from build123d import *

# Parameters (mm, degrees)
SKETCH_1_R          = 2.75
EXTRUDE_1_DEPTH     = 10
CUT_EXTRUDE_1_REACH = 38.009
SKETCH_3_R          = 2.25
SKETCH_3_3_R        = 1.65
CUT_EXTRUDE_2_DEPTH = 37.00893353
FILLET_1_R          = 1
FILLET_2_R          = 0.5
CHAMFER_1_SIZE      = 0.5


with BuildPart() as part:
    # 草图1 → 凸台-拉伸1 (new body)
    with BuildSketch(Plane(origin=(0, 0, 0), x_dir=(1, 0, 0), z_dir=(0, 1, 0))):
        with BuildLine():
            ThreePointArc((5.025690834, 18.234375), (-0.716951035, 21.453070806), (-5.432446466, 16.859375))
            Line((-5.432446466, 16.859375), (-6.517551571, 10))
            Line((-6.517551571, 10), (-14.296618271, 10))
            Line((-14.296618271, 10), (-14.296618271, 0.5))
            Line((-14.296618271, 0.5), (-3.968626967, 0.5))
            ThreePointArc((-3.968626967, 0.5), (4, 0), (-3.968626967, -0.5))
            Line((-3.968626967, -0.5), (-14.296618271, -0.5))
            Line((-14.296618271, -0.5), (-14.296618271, -10))
            Line((-14.296618271, -10), (-6.517551571, -10))
            Line((-6.517551571, -10), (-5.432446466, -16.859375))
            ThreePointArc((-5.432446466, -16.859375), (-0.716951035, -21.453070806), (5.025690834, -18.234375))
            Line((5.025690834, -18.234375), (10.965143638, -4.875))
            ThreePointArc((10.965143638, -4.875), (12, 0), (10.965143638, 4.875))
            Line((10.965143638, 4.875), (5.025690834, 18.234375))
        make_face()
        with Locations(Location((0, -16, 0), (0, 0, 270))):
            Circle(SKETCH_1_R, mode=Mode.SUBTRACT)
        with Locations(Location((0, 16, 0), (0, 0, 270))):
            Circle(SKETCH_1_R, mode=Mode.SUBTRACT)
    extrude(amount=EXTRUDE_1_DEPTH)

    # 草图3 → 切除-拉伸1 (cut, up to next)
    with BuildSketch(Plane.XY.offset(10), mode=Mode.PRIVATE) as cut_extrude_1_sk1:
        with Locations((-10.296618271, 5)):
            Circle(SKETCH_3_R)
    cut_extrude_1_tool1 = extrude(cut_extrude_1_sk1.sketch, amount=-CUT_EXTRUDE_1_REACH, mode=Mode.PRIVATE) & part.part
    add(cut_extrude_1_tool1.solids().sort_by_distance((-10.296618, 5, 10))[0], mode=Mode.SUBTRACT)

    # 草图3<3> → 切除-拉伸2 (cut, through all)
    with BuildSketch(Plane.XY.offset(10)):
        with Locations(Location((-10.296618271, 5, 0), (0, 0, 180))):
            Circle(SKETCH_3_3_R)
    extrude(amount=-CUT_EXTRUDE_2_DEPTH, mode=Mode.SUBTRACT)

    # 圆角1
    fillet_1_edges = [part.edges().sort_by_distance(p)[0] for p in [
        (-14.296618271, 5, 10),
        (-14.296618271, 5, -10),
    ]]
    fillet(fillet_1_edges, radius=FILLET_1_R)

    # 圆角2
    fillet_2_edges = [part.edges().sort_by_distance(p)[0] for p in [
        (-6.517551571, 5, 10),
        (-14.296618271, 5, 0.5),
        (-14.296618271, 5, -0.5),
        (-6.517551571, 5, -10),
    ]]
    fillet(fillet_2_edges, radius=FILLET_2_R)

    # 倒角1
    chamfer_1_edges = [part.edges().sort_by_distance(p)[0] for p in [
        (-6.619913143, 0, 10.119827342),
        (-6.619913143, 10, 10.119827342),
        (-6.619913143, 0, -10.119827342),
        (-6.619913143, 10, -10.119827342),
        (-0.716951035, 10, 21.453070806),
        (7.995417236, 10, 11.5546875),
        (0, 0, 13.25),
        (0, 0, -18.75),
        (4, 0, 0),
        (12, 10, 0),
        (-5.941630183, 0, -13.640625),
        (-0.716951035, 0, -21.453070806),
        (7.995417236, 0, -11.5546875),
        (12, 0, 0),
        (7.995417236, 0, 11.5546875),
        (-0.716951035, 0, 21.453070806),
        (-5.941630183, 0, 13.640625),
        (7.995417236, 10, -11.5546875),
        (-0.716951035, 10, -21.453070806),
        (-5.941630183, 10, -13.640625),
        (4, 10, 0),
        (-14.296618271, 0, -5),
        (-14.296618271, 10, -5),
        (-10.12064547, 0, 10),
        (-10.12064547, 0, -10),
        (-14.003725052, 0, 9.707106781),
        (-14.003725052, 0, -9.707106781),
        (-10.12064547, 10, -10),
        (-5.941630183, 10, 13.640625),
        (-10.12064547, 10, 10),
        (-14.003725052, 10, 9.707106781),
        (-14.003725052, 10, -9.707106781),
        (0, 10, -18.75),
        (-8.882622619, 0, -0.5),
        (-8.882622619, 10, -0.5),
        (0, 10, 13.25),
        (-14.296618271, 0, 5),
        (-8.882622619, 0, 0.5),
        (-14.150171662, 0, 0.646446609),
        (-14.150171662, 0, -0.646446609),
        (-8.882622619, 10, 0.5),
        (-14.296618271, 10, 5),
        (-14.150171662, 10, 0.646446609),
        (-14.150171662, 10, -0.646446609),
    ]]
    chamfer(chamfer_1_edges, length=CHAMFER_1_SIZE - 0.0001)  # a hair under: the kernel refuses the full size


solid = part.part
The model under review builds one solid part; all positions refer to its coordinate system, in mm. A direction names the side the tool comes from. Give positions to 0.01 mm unless a question says otherwise; leave off trailing zeros. Loops run counter-clockwise (first coordinate to the right, second up) from the corner with the lowest first, then second, coordinate; pieces in that order, holes last. Notation, with made-up numbers: (14.5, -6.75) -> (67.5, -6.75) arc R12 cw to (67.5, 9.25) -> close; hole circle Ø4 at (79.25, 51.5). An arc over 180 degrees is marked (long way). Put each result on its own line as item: value. Start each with the question number.
1. For faces 1 (the face through (-4, 0, 4)), 2 (the face through (-7.7, 4.9, 0.5)), 3 (the face through (-8, 4, 10)), list the 3-axis set-ups (+Z, -Z, +X, -X, +Y, -Y) from which the entire face can be reached by the end or side of a thin tool; tool diameter is ignored.
2. Mouldability with a two-part tool opening along X and no side actions: class faces 4 (the face through (-14.297, 5, -5)), 5 (the face through (-8.15, 5.68, 5.32)), 6 (the face through (11.64, 0.14, -0.07)) as released by +X, released by -X, zero draft, split by the parting line, or undercut.
3. Wall thickness on probe 1 along Z at (x, y) = (-9.5, 2.75); probe 2 along Z at (x, y) = (2.25, 7); probe 3 along X at (y, z) = (9, -16): over which ranges is each line inside the solid? List them lowest first.
4. We need section C-C on z = 0. State the section outline as (x, y) points.
5. We need section A-A on y = 5. State how many separate pieces and enclosed holes the cut face has, then the cut area to 3 significant figures.
6. Clearance check with flat-ended pins moving along their axes: P1, Ø6, axis at x = -10.3, y = 5, coming from the +Z side; P2, Ø5, axis at x = 0, z = 0, coming from the -Y side; P3, Ø6, axis at x = 2.5, y = 8.5, coming from the -Z side; P4, Ø5, axis at x = 8.5, y = 4.5, coming from the -Z side. State where each tip first meets the part, or that it passes through.
7. We need section D-D on y = 8.75. State the section outline as (x, z) points (3 decimals), then the cut area to 3 significant figures.
Determined:
1. face 1: +Z, -Z, +X, -X, -Y
1. face 2: -X, +Y, -Y
1. face 3: +Z, -X, +Y, -Y
2. face 4: released by -X
2. face 5: undercut
2. face 6: released by +X
3. probe 1: -10 to -0.5, 0.5 to 10
3. probe 2: -21.02 to -17.58, -14.42 to -3.31, 3.31 to 14.42, 17.58 to 21.02
3. probe 3: -5.57 to -2.75, 2.75 to 6.02
4. outline: (4, 0.5) -> (4.5, 0) -> (11.5, 0) -> (12, 0.5) -> (12, 9.5) -> (11.5, 10) -> (4.5, 10) -> (4, 9.5) -> close
5. separate pieces: 3
5. enclosed holes: 2
5. area: 574 mm^2
6. P1: z = 10
6. P2: through
6. P3: z = -21.5
6. P4: z = -16.04
7. outline: (-14.297, -9) arc R1 ccw to (-13.297, -10) -> (-6.945, -10) arc R0.5 cw to (-6.451, -10.422) -> (-5.432, -16.859) arc R5.5 ccw to (5.026, -18.234) -> (10.965, -4.875) arc R12 ccw to (10.965, 4.875) -> (5.026, 18.234) arc R5.5 ccw to (-5.432, 16.859) -> (-6.451, 10.422) arc R0.5 cw to (-6.945, 10) -> (-13.297, 10) arc R1 ccw to (-14.297, 9) -> (-14.297, 1) arc R0.5 ccw to (-13.797, 0.5) -> (-3.969, 0.5) arc R4 cw (long way) to (-3.969, -0.5) -> (-13.797, -0.5) arc R0.5 ccw to (-14.297, -1) -> close; hole circle Ø5.5 at (0, -16); hole circle Ø5.5 at (0, 16)
7. area: 648 mm^2
